Autodesk Inventor part; units mm, degrees
ref_plane "YZ Plane" through (0, 0, 0) normal (1, 0, 0) x (0, 1, 0)
ref_plane "XZ Plane" through (0, 0, 0) normal (0, 1, 0) x (-1, 0, 0)
ref_plane "XY Plane" through (0, 0, 0) normal (0, 0, 1) x (1, 0, 0)
sketch "Sketch1" plane through (0, 0, 0) normal (0, 1, 0) x (-1, 0, 0)
  line L0 (-0.4496, -30) -> (-0.4496, 0)
  line L1 (-32.1589, 0) -> (-32.1589, -30)
  circle A0 centre (-65.2986, -15) radius 2.55
  circle A1 centre (32.69, -15) radius 2.6
  circle A2 centre (-7.0193, -15) radius 1.05
  circle A3 centre (-14.0193, -8) radius 1.05
  circle A4 centre (-14.0193, -22) radius 1.05
  circle A5 centre (-21.0193, -15) radius 1.05
  circle A6 centre (-14.0193, -15) radius 2.6
  circle A7 centre (25.69, -15) radius 1.05
  circle A8 centre (32.69, -8) radius 1.05
  circle A9 centre (32.69, -22) radius 1.05
  circle A10 centre (39.69, -15) radius 1.05
  line L2 (36.9177, -5.9376) -> (24.19, 0)
  line L3 (-56.7986, 0) -> (-69.5263, -5.9376)
  arc A11 (36.9177, -24.0624) -> (36.9177, -5.9376) centre (32.69, -15) ccw
  line L4 (24.19, -30) -> (36.9177, -24.0624)
  line L5 (-69.5263, -24.0624) -> (-56.7986, -30)
  arc A12 (-69.5263, -5.9376) -> (-69.5263, -24.0624) centre (-65.2986, -15) ccw
  line L6 (-56.7986, 0) -> (24.19, 0)
  line L7 (24.19, -30) -> (-56.7986, -30)
  line L8 (-32.6086, -30) -> (-32.6086, 0)
  line L9 (-31.7093, 0) -> (-31.7093, -30)
  line L10 (-0.8993, -30) -> (-0.8993, 0)
  line L11 (0, 0) -> (0, -30)
  point P0 (0, 0)
extrude "Extrusion1" add sketch "Sketch1" against normal blind 1.5
properties part number "CAM_axis_1_top_frame"
Work out the finished part from the listing and answer in its coordinate system (mm). Coordinates: 2 decimals unless noted, no trailing zeros. Loops run counter-clockwise (first coordinate to the right, second up) from the corner with the lowest first, then second, coordinate; pieces in that order, holes last. Notation, with made-up numbers: (-21, 8.5) -> (38, 8.5) arc R31 ccw to (38, 37.5) -> close; hole circle Ø9 at (34.25, 32). An arc over 180 degrees is marked (long way). Answer as CSV lines item,"result".
1) The part is cut by section B-B (x = -25.69). Give the vertices of the cut face in (y, z).
A:
outline,"(-1.5, -29.3) -> (0, -29.3) -> (0, -16.05) -> (-1.5, -16.05) -> close; (-1.5, -13.95) -> (0, -13.95) -> (0, -0.7) -> (-1.5, -0.7) -> close"
2) The part is cut by section A-A (z = -15). State how many separate pieces and enclosed holes the cut face has, and give its area (3 significant figures).
A:
separate pieces,"8"
enclosed holes,"0"
area,"141 mm²"
3) A flat-ended cylindrical pin translates along its axis: pin 1 (3 mm diameter, centred on x = -32.69, z = -15, fed in from -Y). Find the tip coordinate at first contact, or state that the pin passes through.
A:
pin 1,"passes through"
4) The part is cut by section D-D (z = -22). Give the vertices of the cut face in (x, y), and give its area (3 significant figures).
A:
outline,"(-39.83, -1.5) -> (-33.74, -1.5) -> (-33.74, 0) -> (-39.83, 0) -> close; (-31.64, -1.5) -> (12.97, -1.5) -> (12.97, 0) -> (-31.64, 0) -> close; (15.07, -1.5) -> (72.44, -1.5) -> (72.44, 0) -> (15.07, 0) -> close"
area,"162 mm²"
5) Straight lines are drawn through the part: probe 1 along X at (y, z) = (-0.55, -21.5); probe 2 along X at (y, z) = (-0.85, -28); probe 3 along Z at (x, y) = (63, -1.05). For each, find the intervals that lie inside material, in ascending order.
A:
probe 1,"x = -40.29 to -33.61, -31.77 to 13.1, 14.94 to 72.9"
probe 2,"x = -28.48 to 61.09"
probe 3,"z = -27.11 to -16.1, -13.9 to -2.89"
6) For a pull along Z with two mould halves and no side action, classify faces 1 (the face through (-42.69, -0.74, -15.16)), 2 (the face through (-30.465, -0.74, -27.073)), 3 (the face through (-33.175, -0.74, -22.932)) as released by +Z, released by -Z, zero draft, split by the parting line, or undercut.
A:
face 1,"split by the parting line"
face 2,"released by -Z"
face 3,"undercut"
